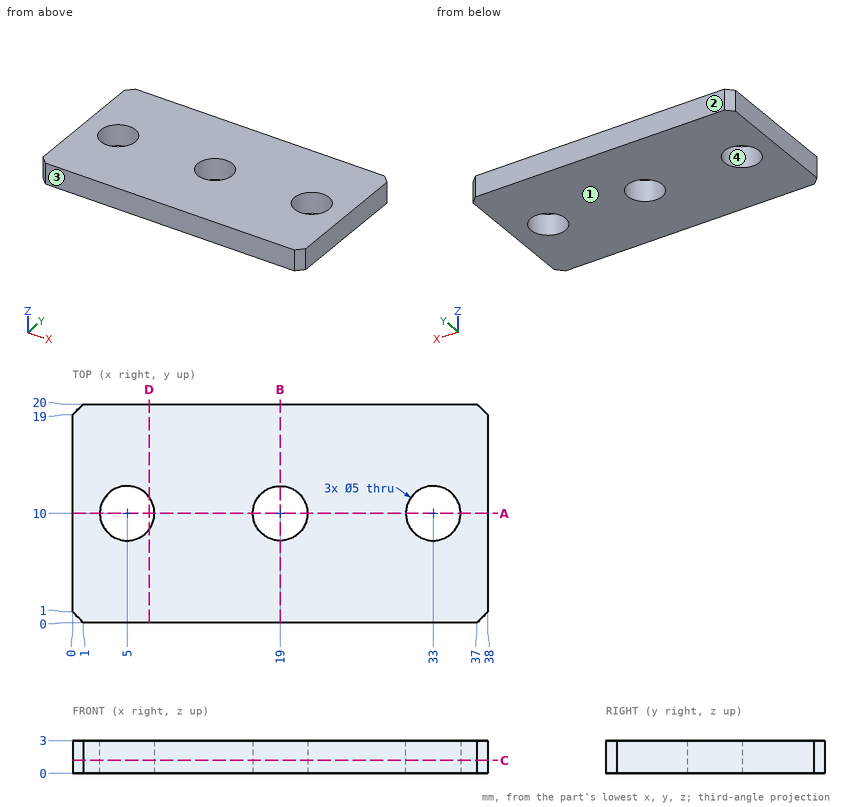
Answer from the drawing. Dimensions are ordinates in mm from the lowest x, y and z of the part. Round coordinates to 2 decimals unless told otherwise and drop trailing zeros. Order: outer loops, then holes, each group sorted by start corner. A loop starts at its lowest first (then second) coordinate and runs counter-clockwise, first axis right, second up.
1) Straight lines are drawn through the part: L1, parallel to Y at x = 19, z = 1; L2, parallel to X at y = 9.5, z = 0.9; L3, parallel to Y at x = 18, z = 0.3. For each, find the intervals that lie inside material, in ascending order.
2) The part is cut by section A-A on y = 10. Write down the section's boundary in (x, z).
3) The part is cut by section B-B on x = 19. Write down the section's boundary in (y, z).
4) The part is cut by section D-D on x = 7. Write down the section's boundary in (y, z).
5) Flat-ended cylindrical pins translate along their axes: pin 1 (12 mm diameter, centred on x = 16.5, y = 6, fed in from -Z); pin 2 (2 mm diameter, centred on x = 18.5, y = 11, fed in from +Z). Find the tip coordinate at first contact, or state that the pin passes through.
6) The part is cut by section C-C on z = 1.2. Write down the section's boundary in (x, y).
7) The mould has two halves that part along Y. Classify the marked faces 1, 2, 3 and 4: released by +Y, released by -Y, zero draft, split by the parting line, or undercut.
Resolved:
1. L1: y = 0 to 7.5, 12.5 to 20
1. L2: x = 0 to 2.55, 7.45 to 16.55, 21.45 to 30.55, 35.45 to 38
1. L3: y = 0 to 7.71, 12.29 to 20
2. outline: (0, 0) - (2.5, 0) - (2.5, 3) - (0, 3) - close; (7.5, 0) - (16.5, 0) - (16.5, 3) - (7.5, 3) - close; (21.5, 0) - (30.5, 0) - (30.5, 3) - (21.5, 3) - close; (35.5, 0) - (38, 0) - (38, 3) - (35.5, 3) - close
3. outline: (0, 0) - (7.5, 0) - (7.5, 3) - (0, 3) - close; (12.5, 0) - (20, 0) - (20, 3) - (12.5, 3) - close
4. outline: (0, 0) - (8.5, 0) - (8.5, 3) - (0, 3) - close; (11.5, 0) - (20, 0) - (20, 3) - (11.5, 3) - close
5. pin 1: stops at z = 0
5. pin 2: passes through
6. outline: (0, 1) - (1, 0) - (37, 0) - (38, 1) - (38, 19) - (37, 20) - (1, 20) - (0, 19) - close; hole circle Ø5 at (5, 10); hole circle Ø5 at (19, 10); hole circle Ø5 at (33, 10)
7. face 1: zero draft
7. face 2: released by +Y
7. face 3: released by -Y
7. face 4: undercut
